from build123d import *

# Parameters (mm, degrees)
SKETCH_1_W          = 72
SKETCH_1_H          = 99
EXTRUDE_1_DEPTH     = 2
SKETCH_3_R          = 1.525
CUT_EXTRUDE_1_DEPTH = 2
SKETCH_4_R          = 1.525
CUT_EXTRUDE_2_DEPTH = 2
SKETCH_5_W          = 32
SKETCH_5_H          = 58
CUT_EXTRUDE_3_DEPTH = 2
FILLET_1_R          = 2
CUT_EXTRUDE_4_DEPTH = 2
FILLET_2_R          = 2


with BuildPart() as part:
    # 草图1 → 凸台-拉伸1 (new body)
    with BuildSketch(Plane(origin=(0, 0, 0), x_dir=(1, 0, 0), z_dir=(0, 1, 0))):
        Rectangle(SKETCH_1_W, SKETCH_1_H)
    extrude(amount=EXTRUDE_1_DEPTH)

    # 草图3 → 切除-拉伸1 (cut)
    with BuildSketch(Plane(origin=(0, 2, 0), x_dir=(1, 0, 0), z_dir=(0, 1, 0))):
        with Locations(Location((33, 46.5, 0), (0, 0, 270))):
            Circle(SKETCH_3_R)
        with Locations(Location((-33, 46.5, 0), (0, 0, 270))):
            Circle(SKETCH_3_R)
        with Locations(Location((-33, -46.5, 0), (0, 0, 270))):
            Circle(SKETCH_3_R)
        with Locations(Location((33, -46.5, 0), (0, 0, 270))):
            Circle(SKETCH_3_R)
    extrude(amount=-CUT_EXTRUDE_1_DEPTH, mode=Mode.SUBTRACT)

    # 草图4 → 切除-拉伸2 (cut)
    with BuildSketch(Plane(origin=(0, 2, 0), x_dir=(1, 0, 0), z_dir=(0, 1, 0))):
        with Locations(Location((16, -32, 0), (0, 0, 270))):
            Circle(SKETCH_4_R)
        with Locations(Location((-16, -32, 0), (0, 0, 270))):
            Circle(SKETCH_4_R)
        with Locations(Location((-16, 32, 0), (0, 0, 270))):
            Circle(SKETCH_4_R)
        with Locations(Location((16, 32, 0), (0, 0, 270))):
            Circle(SKETCH_4_R)
    extrude(amount=-CUT_EXTRUDE_2_DEPTH, mode=Mode.SUBTRACT)

    # 草图5 → 切除-拉伸3 (cut)
    with BuildSketch(Plane(origin=(0, 2, 0), x_dir=(1, 0, 0), z_dir=(0, 1, 0))):
        Rectangle(SKETCH_5_W, SKETCH_5_H)
    extrude(amount=-CUT_EXTRUDE_3_DEPTH, mode=Mode.SUBTRACT)

    # 圆角1
    fillet_1_edges = [part.edges().sort_by_distance(p)[0] for p in [
        (16, 1, -29),
        (16, 1, 29),
        (-16, 1, 29),
        (-16, 1, -29),
    ]]
    fillet(fillet_1_edges, radius=FILLET_1_R)

    # 草图6 → 切除-拉伸4 (cut)
    with BuildSketch(Plane(origin=(0, 2, 0), x_dir=(1, 0, 0), z_dir=(0, 1, 0))):
        with BuildLine():
            Line((22, -28), (22, 28))
            ThreePointArc((22, 28), (25.5, 31.5), (29, 28))
            Line((29, 28), (29, -28))
            ThreePointArc((29, -28), (25.5, -31.5), (22, -28))
        make_face()
        with BuildLine():
            Line((-22, -28), (-22, 28))
            ThreePointArc((-22, 28), (-25.5, 31.5), (-29, 28))
            Line((-29, 28), (-29, -28))
            ThreePointArc((-29, -28), (-25.5, -31.5), (-22, -28))
        make_face()
        with BuildLine():
            Line((-22.5, 43.5), (22.5, 43.5))
            ThreePointArc((22.5, 43.5), (26, 40), (22.5, 36.5))
            Line((22.5, 36.5), (-22.5, 36.5))
            ThreePointArc((-22.5, 36.5), (-26, 40), (-22.5, 43.5))
        make_face()
        with BuildLine():
            Line((-22.5, -43.5), (22.5, -43.5))
            ThreePointArc((22.5, -43.5), (26, -40), (22.5, -36.5))
            Line((22.5, -36.5), (-22.5, -36.5))
            ThreePointArc((-22.5, -36.5), (-26, -40), (-22.5, -43.5))
        make_face()
    extrude(amount=-CUT_EXTRUDE_4_DEPTH, mode=Mode.SUBTRACT)

    # 圆角2
    fillet_2_edges = [part.edges().sort_by_distance(p)[0] for p in [
        (36, 1, 49.5),
        (-36, 1, 49.5),
        (-36, 1, -49.5),
        (36, 1, -49.5),
    ]]
    fillet(fillet_2_edges, radius=FILLET_2_R)


solid = part.part
Read the model definition and answer for the solid it produces. Units are mm, in the model's axes. Coordinates: 2 decimals unless noted, no trailing zeros. Write each loop counter-clockwise with the first axis right and the second up, starting at its lowest first coordinate (ties: lowest second). Pieces come first, ordered by that corner, then holes. Notation, with made-up numbers: (87, -13) -> (104, -13) arc R19 cw to (104, 9) -> close; hole circle Ø4 at (-37, 13). An arc over 180 degrees is marked (long way). Return JSON: item names as keys, results as strings.
(1) The part is cut by section A-A on x = -7. Give the vertices of the cut face in (y, z).
Answers below:
{"outline": "(0, -49.5) -> (2, -49.5) -> (2, -43.5) -> (0, -43.5) -> close; (0, -36.5) -> (2, -36.5) -> (2, -29) -> (0, -29) -> close; (0, 29) -> (2, 29) -> (2, 36.5) -> (0, 36.5) -> close; (0, 43.5) -> (2, 43.5) -> (2, 49.5) -> (0, 49.5) -> close"}
(2) The part is cut by section B-B on z = 46.5. Give the vertices of the cut face in (x, y) (3 decimals).
Answers below:
{"outline": "(-36, 0) -> (-34.525, 0) -> (-34.525, 2) -> (-36, 2) -> close; (-31.475, 0) -> (31.475, 0) -> (31.475, 2) -> (-31.475, 2) -> close; (34.525, 0) -> (36, 0) -> (36, 2) -> (34.525, 2) -> close"}
(3) The part is cut by section C-C on x = 33. Give the vertices of the cut face in (y, z) (3 decimals), then the cut area to 3 significant figures.
Answers below:
{"outline": "(0, -49.5) -> (2, -49.5) -> (2, -48.025) -> (0, -48.025) -> close; (0, -44.975) -> (2, -44.975) -> (2, 44.975) -> (0, 44.975) -> close; (0, 48.025) -> (2, 48.025) -> (2, 49.5) -> (0, 49.5) -> close", "area": "186 mm^2"}
(4) The part is cut by section D-D on z = -13. Give the vertices of the cut face in (x, y), then the cut area to 3 significant figures.
Answers below:
{"outline": "(-36, 0) -> (-29, 0) -> (-29, 2) -> (-36, 2) -> close; (-22, 0) -> (-16, 0) -> (-16, 2) -> (-22, 2) -> close; (16, 0) -> (22, 0) -> (22, 2) -> (16, 2) -> close; (29, 0) -> (36, 0) -> (36, 2) -> (29, 2) -> close", "area": "52.0 mm^2"}
(5) This flat-tipped pin is pushed along its axis until it touches: P1, Ø2.5, axis at x = 33, z = 46.5, coming from the +Y side. Where does it stop, or does it pass through?
Answers below:
{"P1": "through"}
(6) For a pull along X with two mould halves and no side action, classify faces 1 (the flat face through (36, 1, 1)), 2 (the cylindrical face through (32.07, 1.01, -47.71)) as pulls with the +X half, pulls with the -X half, needs draft (parallel to the pull), parting line crosses it, or undercut.
Answers below:
{"face 1": "pulls with the +X half", "face 2": "undercut"}
(7) Consider line 1 along X through (y, z) = (0.8, 46.5) (3 decimals); line 2 along Z through (x, y) = (20.5, 0.2); line 3 along X through (y, z) = (1.6, 32) (3 decimals). Determine where each line is inside the solid, lowest interval first. Write a range as from..to.
Answers below:
{"line 1": "-36..-34.525, -31.475..31.475, 34.525..36", "line 2": "-49.5..-43.5, -36.5..36.5, 43.5..49.5", "line 3": "-36..-17.525, -14.475..14.475, 17.525..36"}
